Source: CAD feature listing. Evaluate the final solid. Frame: model axes, mm. A direction names the side the tool comes from. Round coordinates to 2 decimals unless told otherwise and drop trailing zeros. Loops run counter-clockwise (first coordinate to the right, second up) from the corner with the lowest first, then second, coordinate; pieces in that order, holes last. Notation, with made-up numbers: M -35,4.5 L 1,4.5 A11 ccw 1,24.5 Z; hole C -13,6.5 d5. An arc over 180 degrees is marked long. Answer as CSV lines item,"result". Start each with the question number.
```python
from build123d import *

# Parameters (mm, degrees)
SKETCH1_R           = 0.3048
PINS_DEPTH          = 2.54
PINS_2_DEPTH        = 2.54
PINS_3_DEPTH        = 2.54
PINS_4_DEPTH        = 2.54
PINS_5_DEPTH        = 2.54
PINS_6_DEPTH        = 2.54
SKETCH2_W           = 7.3152
SKETCH2_H           = 10.795
MAIN_BODY_DEPTH     = 8.382
SKETCH3_W           = 1.0922
SKETCH3_H           = 1.524
SKETCH3_H_2         = 1.016
FEET_DEPTH          = 0.635
SKETCH5_W           = 7.3152
SKETCH5_H           = 8.382
BOSS_EXTRUDE5_DEPTH = 3.9878
SKETCH4_R           = 2.54
CUP_DEPTH           = 19.4818
SKETCH6_R           = 2.3495
SPRING_DEPTH        = 6.5532
FILLET1_R           = 0.635


with BuildPart() as part:
    # Sketch1 → Pins (new body)
    with BuildSketch(Plane(origin=(0, 0, 0), x_dir=(1, 0, 0), z_dir=(0, 1, 0))):
        with Locations(Location((0, 0, 0), (0, 0, 270))):
            Circle(SKETCH1_R)
    extrude(amount=-PINS_DEPTH)



with BuildPart() as body_2:
    # Sketch1 → Pins 2 (new body)
    with BuildSketch(Plane(origin=(0, 0, 0), x_dir=(1, 0, 0), z_dir=(0, 1, 0))):
        with Locations(Location((0, -2.4892, 0), (0, 0, 270))):
            Circle(SKETCH1_R)
    extrude(amount=-PINS_2_DEPTH)


with BuildPart() as body_3:
    # Sketch1 → Pins 3 (new body)
    with BuildSketch(Plane(origin=(0, 0, 0), x_dir=(1, 0, 0), z_dir=(0, 1, 0))):
        with Locations(Location((0, -4.9784, 0), (0, 0, 270))):
            Circle(SKETCH1_R)
    extrude(amount=-PINS_3_DEPTH)


with BuildPart() as body_4:
    # Sketch1 → Pins 4 (new body)
    with BuildSketch(Plane(origin=(0, 0, 0), x_dir=(1, 0, 0), z_dir=(0, 1, 0))):
        with Locations(Location((2.5146, 0, 0), (0, 0, 270))):
            Circle(SKETCH1_R)
    extrude(amount=-PINS_4_DEPTH)


with BuildPart() as body_5:
    # Sketch1 → Pins 5 (new body)
    with BuildSketch(Plane(origin=(0, 0, 0), x_dir=(1, 0, 0), z_dir=(0, 1, 0))):
        with Locations(Location((2.5146, -2.4892, 0), (0, 0, 270))):
            Circle(SKETCH1_R)
    extrude(amount=-PINS_5_DEPTH)


with BuildPart() as body_6:
    # Sketch1 → Pins 6 (new body)
    with BuildSketch(Plane(origin=(0, 0, 0), x_dir=(1, 0, 0), z_dir=(0, 1, 0))):
        with Locations(Location((2.5146, -4.9784, 0), (0, 0, 270))):
            Circle(SKETCH1_R)
    extrude(amount=-PINS_6_DEPTH)


with BuildPart() as part_1:
    add(part.part)

    add(body_2.part)  # Main Body merges body 2

    add(body_3.part)  # Main Body merges body 3

    add(body_4.part)  # Main Body merges body 4

    add(body_5.part)  # Main Body merges body 5

    add(body_6.part)  # Main Body merges body 6
    # Sketch2 → Main Body (add)
    with BuildSketch(Plane(origin=(0, 0, 0), x_dir=(1, 0, 0), z_dir=(0, 1, 0))):
        with Locations((1.2573, -3.1877)):
            Rectangle(SKETCH2_W, SKETCH2_H)
    extrude(amount=MAIN_BODY_DEPTH)

    # Sketch3 → Feet (add)
    with BuildSketch(Plane.XZ):
        with Locations((-1.8542, 7.8232)):
            Rectangle(SKETCH3_W, SKETCH3_H)
        with Locations((4.3688, 7.8232)):
            Rectangle(SKETCH3_W, SKETCH3_H)
        with Locations((4.3688, -1.7018)):
            Rectangle(SKETCH3_W, SKETCH3_H_2)
        with Locations((-1.8542, -1.7018)):
            Rectangle(SKETCH3_W, SKETCH3_H_2)
    extrude(amount=FEET_DEPTH)

    # Sketch5 → Boss-Extrude5 (add)
    with BuildSketch(Plane(origin=(0, 0, -2.2098), x_dir=(-1, 0, 0), z_dir=(0, 0, -1))):
        with Locations((-1.2573, 4.191)):
            Rectangle(SKETCH5_W, SKETCH5_H)
    extrude(amount=BOSS_EXTRUDE5_DEPTH)

    # Sketch4 → Cup (add)
    with BuildSketch(Plane(origin=(0, 0, -2.2098), x_dir=(-1, 0, 0), z_dir=(0, 0, -1))):
        with Locations((-1.2573, 4.3688)):
            Circle(SKETCH4_R)
    extrude(amount=CUP_DEPTH)

    # Sketch6 → Spring (add)
    with BuildSketch(Plane(origin=(0, 0, -6.1976), x_dir=(-1, 0, 0), z_dir=(0, 0, -1))):
        with Locations((-1.2573, 4.3688)):
            Circle(SKETCH6_R)
    extrude(amount=SPRING_DEPTH)

    # Fillet1
    fillet1_edges = [part_1.edges().sort_by_distance(p)[0] for p in [
        (3.7973, 4.3688, -21.6916),
    ]]
    fillet(fillet1_edges, radius=FILLET1_R)


solid = part_1.part
```
1) Ray query, line 1 along Z through (x, y) = (2.75, -0.75); line 2 along Y through (x, z) = (2.25, -2); line 3 along Z through (x, y) = (-1.5, 6.5). Return the intervals inside material, ascending.
2) Section B-B, the plane z = -5.5. Return loops of the section in (x, y).
3) Access query for faces 5 (the flat face through (-2.4, 4, 1)), 6 (the cylindrical face through (1.588, 6.887, -13.523)). Directions: +Z, -Z, +X, -X, +Y, -Y. A direction counts if a zero-diameter tool reaches every point of the face in a straight line with its end or side. Return the directions, or none.
4) Mould query, pull axis Z, two halves, no side actions, for faces 1 (the flat face through (1, 4, 8.585)), 2 (the flat face through (1, 0, 1)), 3 (the flat face through (4.915, 4, 1)), 4 (the flat face through (1, 4, -21.692)). Classes: pulls with the +Z half, pulls with the -Z half, needs draft (parallel to the pull), parting line crosses it, or undercut.
5) Section A-A, the plane z = 0. Return loops of the section in (x, y).
6) Section C-C, the plane z = -9. Return loops of the section in (x, y).
7) Contact query for flat-ended pins moving along their axis: pin 1 Ø0.5 at (x, z) = (4, 8) entering from -Y (3 decimals); pin 2 Ø4 at (x, z) = (0, -5) entering from -Y. Output: stop coordinate, or through.
Findings below:
1,line 1,"-0.19 to 0.19, 2.3 to 2.68, 4.78 to 5.17"
1,line 2,"0 to 8.38"
1,line 3,"-6.2 to 8.59"
2,outline,"M -2.4,0 L 4.91,0 L 4.91,8.38 L -2.4,8.38 Z"
3,face 5,"+Z, -Z, -X, +Y, -Y"
3,face 6,"-Z"
4,face 1,"pulls with the +Z half"
4,face 2,"undercut"
4,face 3,"needs draft"
4,face 4,"pulls with the -Z half"
5,outline,"M -2.4,0 L -0.3,0 L -0.3,-2.54 L 0.3,-2.54 L 0.3,0 L 2.21,0 L 2.21,-2.54 L 2.82,-2.54 L 2.82,0 L 4.91,0 L 4.91,8.38 L -2.4,8.38 Z"
6,outline,"C 1.26,4.37 d5.08"
7,pin 1,"y = -0.635"
7,pin 2,"y = 0"
